For this review, use the dimensioned drawing (mm, ordinates from the lowest corner) and the shaded views. A direction names the side the tool comes from. Round coordinates to 2 decimals unless told otherwise and drop trailing zeros. Order: outer loops, then holes, each group sorted by start corner. A loop starts at its lowest first (then second) coordinate and runs counter-clockwise, first axis right, second up. Notation, with made-up numbers: (12, -14) - (28, -14) arc R19 ccw to (28, 12) - close; hole circle Ø2 at (14, 7.5). An arc over 180 degrees is marked (long way). Write item = value, one per line.
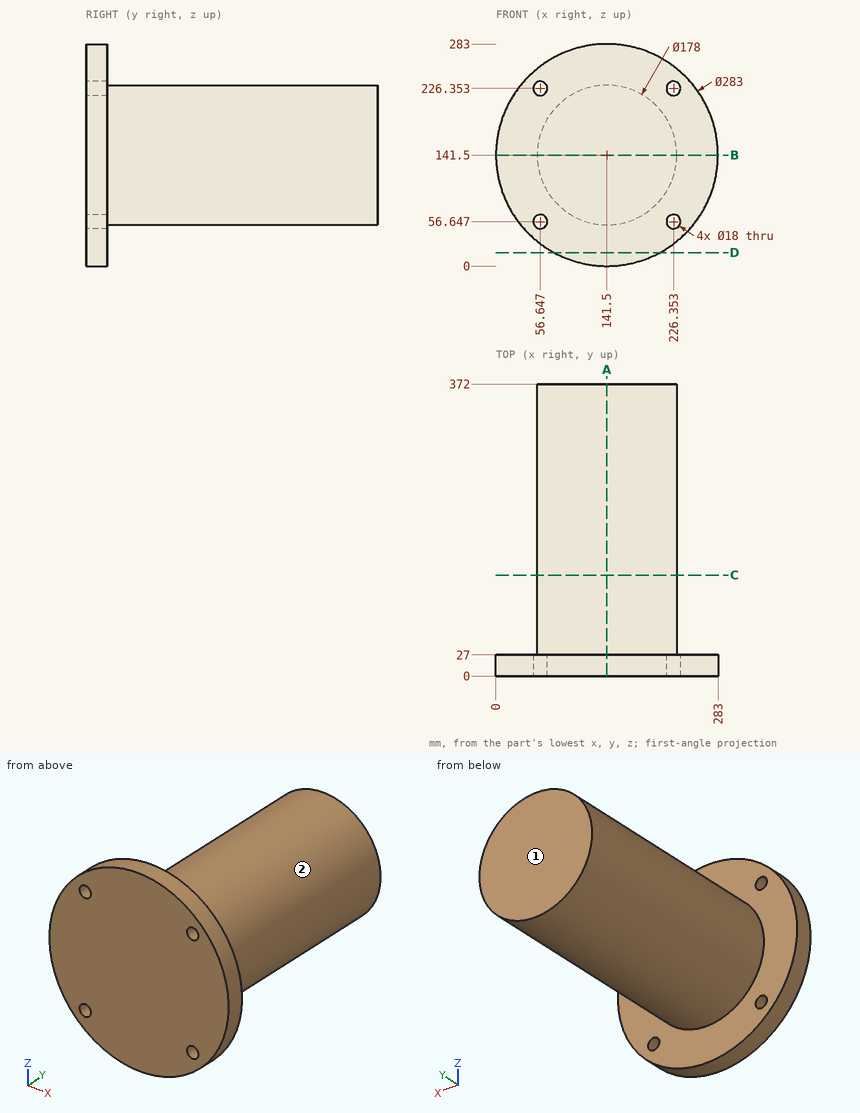
1) Clearance check with flat-ended pins moving along their axes: pin 1 Ø16 at (x, z) = (226.35, 56.65) entering from -Y; pin 2 Ø8 at (x, z) = (65.5, 243) entering from +Y; pin 3 Ø4 at (y, z) = (105.5, 175) entering from +X; pin 4 Ø6 at (x, y) = (62, 84) entering from -Z. State where each tip first meets the part, or that it passes through.
Findings:
pin_1 = through
pin_2 = 27
pin_3 = 224.74
pin_4 = 96.02
2) We need section C-C on y = 128.5. Write out the cut boundary in (x, z), and give its area (3 significant figures).
Findings:
outline = circle Ø178 at (141.5, 141.5)
area = 24,900 mm^2
3) We need section A-A on x = 141.5. Write out the cut boundary in (y, z).
Findings:
outline = (0, 0) - (27, 0) - (27, 52.5) - (372, 52.5) - (372, 230.5) - (27, 230.5) - (27, 283) - (0, 283) - close
4) To check wall thickness, follow L1, parallel to Z at x = 146.5, y = 20.5; L2, parallel to Y at x = 45, z = 133; L3, parallel to X at y = 131, z = 137.5. State the ranges of each line that lie inside material, in increasing order. Write a range as from..to.
Findings:
L1 = 0.09..282.91
L2 = 0..27
L3 = 52.59..230.41
5) For the marked faces 1 and 2, list the 3-axis set-ups (+Z, -Z, +X, -X, +Y, -Y) from which the entire face can be reached by the end or side of a thin tool; tool diameter is ignored.
Findings:
face_1 = +Z, -Z, +X, -X, +Y
face_2 = +Y
6) We need section B-B on z = 141.5. Write out the cut boundary in (x, y), and give its area (3 significant figures).
Findings:
outline = (0, 0) - (283, 0) - (283, 27) - (230.5, 27) - (230.5, 372) - (52.5, 372) - (52.5, 27) - (0, 27) - close
area = 69,100 mm^2
7) We need section D-D on z = 17. Write out the cut boundary in (x, y).
Findings:
outline = (74.25, 0) - (208.75, 0) - (208.75, 27) - (74.25, 27) - close
